from build123d import *

# Parameters (mm, degrees)
SKETCH_1_W          = 65
SKETCH_1_H          = 56
EXTRUDE_1_DEPTH     = 6
SKETCH_2_R          = 1.35
CUT_EXTRUDE_1_DEPTH = 6
FILLET_2_R          = 2
SKETCH_5_R          = 1.6
CUT_EXTRUDE_3_DEPTH = 6
SKETCH_7_R          = 1.6
CUT_EXTRUDE_4_DEPTH = 6
SKETCH_8_R          = 5
CUT_EXTRUDE_5_DEPTH = 6
SKETCH_9_W          = 18
SKETCH_9_H          = 6.5
CUT_EXTRUDE_6_DEPTH = 6
SKETCH_10_W         = 10
SKETCH_10_H         = 5
CUT_EXTRUDE_7_DEPTH = 6
FILLET_3_R          = 2


with BuildPart() as part:
    # 草图1 → 凸台-拉伸1 (new body)
    with BuildSketch(Plane(origin=(0, 0, 0), x_dir=(1, 0, 0), z_dir=(0, 1, 0))):
        Rectangle(SKETCH_1_W, SKETCH_1_H)
    extrude(amount=EXTRUDE_1_DEPTH)

    # 草图2 → 切除-拉伸1 (cut)
    with BuildSketch(Plane(origin=(0, 6, 0), x_dir=(1, 0, 0), z_dir=(0, 1, 0))):
        with Locations(Location((-29, 24.5, 0), (0, 0, 270))):
            Circle(SKETCH_2_R)
        with Locations(Location((29, 24.5, 0), (0, 0, 90))):
            Circle(SKETCH_2_R)
        with Locations(Location((29, -24.5, 0), (0, 0, 270))):
            Circle(SKETCH_2_R)
        with Locations(Location((-29, -24.5, 0), (0, 0, 90))):
            Circle(SKETCH_2_R)
    extrude(amount=-CUT_EXTRUDE_1_DEPTH, mode=Mode.SUBTRACT)

    # 圆角2
    fillet_2_edges = [part.edges().sort_by_distance(p)[0] for p in [
        (32.5, 3, 28),
        (-32.5, 3, 28),
        (-32.5, 3, -28),
        (32.5, 3, -28),
    ]]
    fillet(fillet_2_edges, radius=FILLET_2_R)

    # 草图5 → 切除-拉伸3 (cut)
    with BuildSketch(Plane(origin=(0, 6, 0), x_dir=(1, 0, 0), z_dir=(0, 1, 0))):
        with Locations(Location((-27.5, 13, 0), (0, 0, 270))):
            Circle(SKETCH_5_R)
        with Locations(Location((-3.5, 13, 0), (0, 0, 90))):
            Circle(SKETCH_5_R)
        with Locations(Location((-27.5, -10, 0), (0, 0, 270))):
            Circle(SKETCH_5_R)
        with Locations(Location((-3.5, -10, 0), (0, 0, 90))):
            Circle(SKETCH_5_R)
    extrude(amount=-CUT_EXTRUDE_3_DEPTH, mode=Mode.SUBTRACT)

    # 草图7 → 切除-拉伸4 (cut)
    with BuildSketch(Plane(origin=(0, 6, 0), x_dir=(1, 0, 0), z_dir=(0, 1, 0))):
        with Locations(Location((16.5, 21.59, 0), (0, 0, 270))):
            Circle(SKETCH_7_R)
        with Locations(Location((16.5, -21.59, 0), (0, 0, 90))):
            Circle(SKETCH_7_R)
    extrude(amount=-CUT_EXTRUDE_4_DEPTH, mode=Mode.SUBTRACT)

    # 草图8 → 切除-拉伸5 (cut)
    with BuildSketch(Plane(origin=(0, 6, 0), x_dir=(1, 0, 0), z_dir=(0, 1, 0))):
        with Locations(Location((-12.5, -20, 0), (0, 0, 270))):
            Circle(SKETCH_8_R)
    extrude(amount=-CUT_EXTRUDE_5_DEPTH, mode=Mode.SUBTRACT)

    # 草图9 → 切除-拉伸6 (cut)
    with BuildSketch(Plane(origin=(0, 6, 0), x_dir=(1, 0, 0), z_dir=(0, 1, 0))):
        with Locations((-15.5, 14.75)):
            Rectangle(SKETCH_9_W, SKETCH_9_H)
    extrude(amount=-CUT_EXTRUDE_6_DEPTH, mode=Mode.SUBTRACT)

    # 草图10 → 切除-拉伸7 (cut)
    with BuildSketch(Plane(origin=(0, 6, 0), x_dir=(1, 0, 0), z_dir=(0, 1, 0))):
        with Locations((-19.5, 25.5)):
            Rectangle(SKETCH_10_W, SKETCH_10_H)
    extrude(amount=-CUT_EXTRUDE_7_DEPTH, mode=Mode.SUBTRACT)

    # 圆角3
    fillet_3_edges = [part.edges().sort_by_distance(p)[0] for p in [
        (-14.5, 3, -23),
        (-14.5, 3, -28),
        (-24.5, 3, -28),
        (-24.5, 3, -23),
    ]]
    fillet(fillet_3_edges, radius=FILLET_3_R)


solid = part.part
Input: part model. Units: mm. Frame: model coordinates. A direction names the side the tool comes from. Give positions to 0.01 mm unless a question says otherwise; leave off trailing zeros. Order: outer loops, then holes, each group sorted by start corner. A loop starts at its lowest first (then second) coordinate and runs counter-clockwise, first axis right, second up. Notation, with made-up numbers: M 12,69.5 L 33,69.5 A12 ccw 33,81.5 Z; hole C 15.25,75.25 d11. An arc over 180 degrees is marked long. Answer as a JSON object with one key per item and string values.
1. Pull-direction query (Z, two-part tool) for faces 1 (the flat face through (-16, 3, -11.5)), 2 (the cylindrical face through (-15.1, 2.96, -23.57)), 3 (the cylindrical face through (-26.42, 3.04, -14.18)), 4 (the flat face through (0, 6, 0)); classes: +Z half, -Z half, draft (parallel to the pull), parting line (faces both ways), or undercut.
Result sheet:
{"face 1": "undercut", "face 2": "-Z half", "face 3": "undercut", "face 4": "draft"}
2. Cut plane D-D, the plane z = -21.59. Output: boundary loops of the cut face in (x, y).
Result sheet:
{"outline": "M -32.5,0 L 14.9,0 L 14.9,6 L -32.5,6 Z; M 18.1,0 L 32.5,0 L 32.5,6 L 18.1,6 Z"}
3. Ray query, line 1 (Z direction, x = -22, y = 3); line 2 (X direction, y = 2.95, z = 10); line 3 (X direction, y = 3.5, z = 24). Return the intervals inside material, ascending. Write a range as [from, to].
Result sheet:
{"line 1": "[-23, -18], [-11.5, 28]", "line 2": "[-32.5, -29.1], [-25.9, -5.1], [-1.9, 32.5]", "line 3": "[-32.5, -30.25], [-27.75, -15.5], [-9.5, 27.75], [30.25, 32.5]"}
4. Cut plane A-A, the plane z = 10. Output: boundary loops of the cut face in (x, y).
Result sheet:
{"outline": "M -32.5,0 L -29.1,0 L -29.1,6 L -32.5,6 Z; M -25.9,0 L -5.1,0 L -5.1,6 L -25.9,6 Z; M -1.9,0 L 32.5,0 L 32.5,6 L -1.9,6 Z"}
5. Cut plane B-B, the plane x = -3.5. Output: boundary loops of the cut face in (y, z).
Result sheet:
{"outline": "M 0,-28 L 6,-28 L 6,-14.6 L 0,-14.6 Z; M 0,-11.4 L 6,-11.4 L 6,8.4 L 0,8.4 Z; M 0,11.6 L 6,11.6 L 6,28 L 0,28 Z"}
6. Cut plane C-C, the plane y = 5.1. State how many separate pieces and enclosed holes the cut face has, and give its area (3 significant figures).
Result sheet:
{"separate pieces": "1", "enclosed holes": "12", "area": "3,320 mm²"}
7. Reachability of faces 5 (the flat face through (-16, 3, -18)), 6 (the cylindrical face through (-25.1, 2.96, -27.43)), 7 (the cylindrical face through (31.9, 3.04, 27.43)) from +Z, -Z, +X, -X, +Y, -Y: full face, straight path, thin tool, end or side. Return the list, or none.
Result sheet:
{"face 5": "+Y, -Y", "face 6": "-Z, +Y, -Y", "face 7": "+Z, +X, +Y, -Y"}
8. First-contact query: P1, Ø1, axis at x = 13, z = 18.5, coming from the -Y side. Flat tip, straight axial feed; report the tip coordinate or a pass-through.
Result sheet:
{"P1": "y = 0"}
